Geometry: final body of the model. Coordinates: model frame, mm. Face numbers are marked on the shaded views. A direction names the side the tool comes from. Coordinates: 2 decimals unless noted, no trailing zeros. Write each loop counter-clockwise with the first axis right and the second up, starting at its lowest first coordinate (ties: lowest second). Pieces come first, ordered by that corner, then holes.
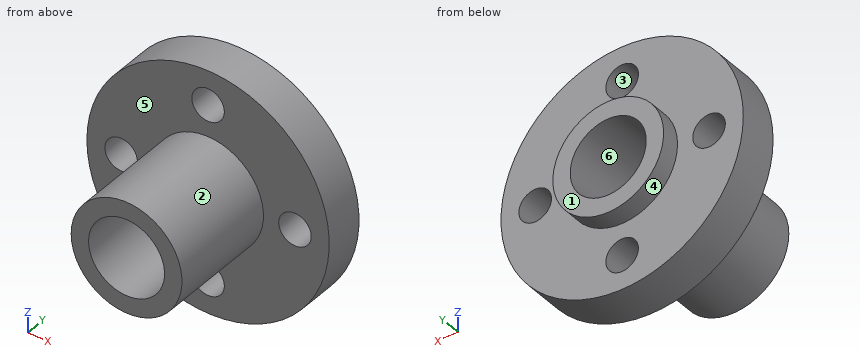
Autodesk Inventor part; units mm, degrees
ref_plane "YZ Plane" through (0, 0, 0) normal (1, 0, 0) x (0, 1, 0)
ref_plane "XZ Plane" through (0, 0, 0) normal (0, 1, 0) x (-1, 0, 0)
ref_plane "XY Plane" through (0, 0, 0) normal (0, 0, 1) x (1, 0, 0)
sketch "Sketch1" plane through (0, 0, 0) normal (0, 1, 0) x (-1, 0, 0)
  circle A0 centre (0, 0) radius 11.15
  circle A1 centre (0, 0) radius 3.5
  circle A2 centre (8, 0) radius 1.5
  line L0 (8, 0) -> (0, 0) construction
  circle A3 centre (0, 8) radius 1.5
  circle A4 centre (-8, 0) radius 1.5
  circle A5 centre (0, -8) radius 1.5
  circle A6 centre (0, 0) radius 5.1
  dimension "d0" = 22.3
  dimension "d1" = 7
  dimension "d2" = 3
  dimension "d3" = 8
  dimension "d6" = 360
  dimension "d8" = 10.2
extrude "Extrusion1" add sketch "Sketch1" along normal blind 3.75 contours A0 | A6
extrude "Extrusion2" add sketch "Sketch1" along normal blind 1.75 from surface at 3.75 contours A6
extrude "Extrusion3" add sketch "Sketch1" against normal blind 10.25 contours A6
properties part number "Leadscrew"
Item 1: Section B-B, the plane y = 1.75. Output: boundary loops of the cut face in (x, z).
Derived:
outline: circle Ø22.3 at (0, 0); hole circle Ø3 at (-8, 0); hole circle Ø7 at (0, 0); hole circle Ø3 at (0, -8); hole circle Ø3 at (0, 8); hole circle Ø3 at (8, 0)
Item 2: Pull-direction query (X, two-part tool) for the marked faces 1, 2 and 3; classes: released by +X, released by -X, zero draft, split by the parting line, or undercut.
Derived:
face 1: zero draft
face 2: split by the parting line
face 3: undercut
Item 3: Set-up query: the marked faces 4, 5 and 6. Return all of +Z, -Z, +X, -X, +Y, -Y with unobstructed straight access to the full face (end or side cutting, diameter ignored); none if empty.
Derived:
face 4: +Y
face 5: -Y
face 6: +Y, -Y
Item 4: Pin query (flat end, axial travel): pin 1 (5 mm diameter, centred on x = 8, z = 0, fed in from +Y); pin 2 (1 mm diameter, centred on y = 0, z = 5, fed in from +X); pin 3 (4 mm diameter, centred on x = 4, y = 2.5, fed in from +Z). Return the tip coordinate at first contact, or that it passes through.
Derived:
pin 1: stops at y = 3.75
pin 2: stops at x = 10.2
pin 3: stops at z = 10.97
Item 5: Section C-C, the plane x = 0. Output: boundary loops of the cut face in (y, z).
Derived:
outline: (-10.25, -5.1) - (0, -5.1) - (0, -6.5) - (3.75, -6.5) - (3.75, -5.1) - (5.5, -5.1) - (5.5, -3.5) - (-10.25, -3.5) - close; (-10.25, 3.5) - (5.5, 3.5) - (5.5, 5.1) - (3.75, 5.1) - (3.75, 6.5) - (0, 6.5) - (0, 5.1) - (-10.25, 5.1) - close; (0, -11.15) - (3.75, -11.15) - (3.75, -9.5) - (0, -9.5) - close; (0, 9.5) - (3.75, 9.5) - (3.75, 11.15) - (0, 11.15) - close
Item 6: Section D-D, the plane x = -8. Output: boundary loops of the cut face in (y, z), plus the area to 3 significant figures.
Derived:
outline: (0, -7.77) - (3.75, -7.77) - (3.75, -1.5) - (0, -1.5) - close; (0, 1.5) - (3.75, 1.5) - (3.75, 7.77) - (0, 7.77) - close
area: 47.0 mm2
Item 7: Section A-A, the plane z = 0. Output: boundary loops of the cut face in (x, y).
Derived:
outline: (-11.15, 0) - (-9.5, 0) - (-9.5, 3.75) - (-11.15, 3.75) - close; (-6.5, 0) - (-5.1, 0) - (-5.1, -10.25) - (-3.5, -10.25) - (-3.5, 5.5) - (-5.1, 5.5) - (-5.1, 3.75) - (-6.5, 3.75) - close; (3.5, -10.25) - (5.1, -10.25) - (5.1, 0) - (6.5, 0) - (6.5, 3.75) - (5.1, 3.75) - (5.1, 5.5) - (3.5, 5.5) - close; (9.5, 0) - (11.15, 0) - (11.15, 3.75) - (9.5, 3.75) - close
Item 8: Material intervals for probe 1 along Z at (x, y) = (0, 1.1); probe 2 along Y at (x, z) = (1.5, 9.25); probe 3 along Z at (x, y) = (-8, 1.85), sorted ascending.
Derived:
probe 1: z = -11.15 to -9.5, -6.5 to -3.5, 3.5 to 6.5, 9.5 to 11.15
probe 2: y = 0 to 3.75
probe 3: z = -7.77 to -1.5, 1.5 to 7.77
